Autodesk Fusion 360 part; units mm, degrees
sketch "Sketch1" plane through (0, 0, 0) normal (0, 0, 1) x (1, 0, 0)
  line L0 (27.5, 28) -> (-37.5, 28)
  line L1 (-37.5, 39) -> (-37.5, -23.5)
  line L2 (-37.5, -28) -> (27.5, -28)
  line L3 (27.5, -28) -> (27.5, 28)
  line L4 (27.5, 23.5) -> (-37.5, 23.5)
  line L5 (-37.5, -23.5) -> (27.5, -23.5)
  line L6 (27.5, -23.5) -> (27.5, 23.5)
  line L7 (27.5, 39) -> (-37.5, 39)
  line L8 (37.5, -28) -> (37.5, 36.48)
  line L9 (27.5, 39) -> (37.5, 36.48)
  line L10 (1.75, 0) -> (22.5, 0)
  line L11 (37.5, 28) -> (37.5, -36.48)
  line L12 (27.5, -39) -> (37.5, -36.48)
  line L13 (27.5, -39) -> (-37.5, -39)
  line L14 (-37.5, -39) -> (-37.5, 23.5)
  dimension "d1" = 65
  dimension "d2" = 56
  dimension "d3" = 65
  dimension "d4" = 47
  dimension "d5" = 11
  dimension "d6" = 10
extrude "Extrude1" add sketch "Sketch1" along normal blind 5.8 contours L0 L1 L3 L4 | L0 L1 L2 L3 L6 L7 L8 L9 L11 L12 L13 L14 | L2 L3 L5 L14
extrude "Extrude2" add sketch "Sketch1" along normal blind 17 contours L0 L1 L2 L3 L6 L7 L8 L9 L11 L12 L13 L14
extrude "Extrude3" add sketch "Sketch1" along normal blind 21 and the other way blind -17
sketch "Sketch2" plane through (0, 0, 21) normal (0, 0, 1) x (-1, 0, 0)
  line L0 (37.5, -39) -> (37.5, 39)
  line L1 (37.5, 39) -> (-27.5, 39)
  line L2 (-27.5, 39) -> (-37.5, 36.48)
  line L3 (-37.5, 36.48) -> (-37.5, -36.48)
  line L4 (-37.5, -36.48) -> (-27.5, -39)
  line L5 (-27.5, -39) -> (37.5, -39)
  circle A0 centre (25, 15) radius 1.5
  circle A1 centre (-15, 15) radius 1.5
  line L6 (-1.75, 0) -> (-22.5, 0)
  circle A2 centre (25, -15) radius 1.5
  circle A3 centre (-15, -15) radius 1.5
  dimension "d15" = 3
  dimension "d16" = 3
extrude "Extrude4" cut sketch "Sketch2" against normal blind 5 contours A0 | A1 | A2 | A3
chamfer "Chamfer1" distance 1 angle 45 4 edges at (-23.6015, 15.5424, 17) (-23.6015, -14.4576, 17) (16.3985, -14.4576, 17) (16.3985, 15.5424, 17)
Here's how the part is built. I have some questions about the finished solid (model axes, mm). A direction names the side the tool comes from. Coordinates: 2 decimals unless noted, no trailing zeros. Write each loop counter-clockwise with the first axis right and the second up, starting at its lowest first coordinate (ties: lowest second). Pieces come first, ordered by that corner, then holes.
1) Thinking about a two-plate mould opening in Y: for faces 1 (the face through (32.43, 37.758, 10.353)), 2 (the face through (-5, -23.5, 3)), 3 (the face through (-5, -39, 10)), which applies, +Y half, -Y half, draft (parallel to the pull), parting line (faces both ways), or undercut?
Filled in:
face 1: +Y half
face 2: undercut
face 3: -Y half
2) I'm going to push flat-ended pins straight in: pin 1 (2.5 mm diameter, centred on x = -25, y = -15, fed in from +Z); pin 2 (8.5 mm diameter, centred on y = 5.5, z = 9.5, fed in from -X). Where does each tip first touch, or does it pass through?
Filled in:
pin 1: passes through
pin 2: stops at x = 27.5
3) If we section it at B-B (y = 15): List the corners of the cut face in (x, z) for me.
Filled in:
outline: (-37.5, 17) - (-27.5, 17) - (-26.5, 18) - (-26.5, 21) - (-37.5, 21) - close; (-23.5, 18) - (-22.5, 17) - (12.5, 17) - (13.5, 18) - (13.5, 21) - (-23.5, 21) - close; (16.5, 18) - (17.5, 17) - (27.5, 17) - (27.5, 0) - (37.5, 0) - (37.5, 21) - (16.5, 21) - close
4) If we section it at C-C (y = 25.5): List the corners of the cut face in (x, z) for me.
Filled in:
outline: (-37.5, 0) - (37.5, 0) - (37.5, 21) - (-37.5, 21) - (-37.5, 17) - (27.5, 17) - (27.5, 5.8) - (-37.5, 5.8) - close
5) If we section it at D-D (x = 24): List the corners of the cut face in (y, z) for me.
Filled in:
outline: (-39, 0) - (-23.5, 0) - (-23.5, 5.8) - (-28, 5.8) - (-28, 17) - (28, 17) - (28, 5.8) - (23.5, 5.8) - (23.5, 0) - (39, 0) - (39, 21) - (-39, 21) - close
6) If we section it at A-A (x = 15): List the corners of the cut face in (y, z) for me, plus the area to 3 significant figures.
Filled in:
outline: (-39, 0) - (-23.5, 0) - (-23.5, 5.8) - (-28, 5.8) - (-28, 17) - (-17.5, 17) - (-16.5, 18) - (-16.5, 21) - (-39, 21) - close; (-13.5, 18) - (-12.5, 17) - (12.5, 17) - (13.5, 18) - (13.5, 21) - (-13.5, 21) - close; (16.5, 18) - (17.5, 17) - (28, 17) - (28, 5.8) - (23.5, 5.8) - (23.5, 0) - (39, 0) - (39, 21) - (16.5, 21) - close
area: 712 mm2
7) If I drill on line 1 (X direction, y = 15, z = 19.45); line 2 (Y direction, x = 15, z = 19.1); line 3 (Z direction, x = -15.5, y = -26), over which ranges is the centre line in solid material (lowest first)?
Filled in:
line 1: x = -37.5 to -26.5, -23.5 to 13.5, 16.5 to 37.5
line 2: y = -39 to -16.5, -13.5 to 13.5, 16.5 to 39
line 3: z = 0 to 5.8, 17 to 21
8) Which directions (+Z, -Z, +X, -X, +Y, -Y) give clear straight access to the entire face, cutting with the end or side of a thin tool? Please do faces 4 (the face through (-5, 0, 17)), 5 (the face through (-1, 27, 0)).
Filled in:
face 4: -X
face 5: -Z, +X, -X, +Y, -Y
